Design review of the part built by this model. Coordinates are the model's own, in mm. A direction names the side the tool comes from. Coordinates: 2 decimals unless noted, no trailing zeros. Order: outer loops, then holes, each group sorted by start corner. A loop starts at its lowest first (then second) coordinate and runs counter-clockwise, first axis right, second up. Notation, with made-up numbers: (63, -21.5) - (84, -21.5) arc R23 cw to (84, 17.5) - close; hole circle Ø2 at (-33, 50.5). An arc over 180 degrees is marked (long way). Write each question's results on one line, items separated by ' | '. Start each with the question number.
```python
from build123d import *

# Parameters (mm, degrees)
F1_W      = 50.8
F1_H      = 50.8
F2_DEPTH  = 508
F5_W      = 50.8
F5_H      = 50.8
F6_DEPTH  = 50.8
F8_W      = 552.45
F8_H      = 552.45
F8_W_2    = 546.1
F8_H_2    = 546.1
F9_DEPTH  = 50.8
F10_DEPTH = 457.2
F12_DEPTH = 114.3
F13_R     = 5.08


# Not quite as in the source:
# - a pattern or mirror of a feature is missing from the dataset's text; its kind, count and spacing are read off the source's solid


with BuildPart() as f2:
    # F1 (on Top) → F2 (new body)
    with BuildSketch(Plane.XY):
        with Locations((-247.65, 247.65)):
            Rectangle(F1_W, F1_H)
    extrude(amount=F2_DEPTH)


with BuildPart() as f3_1:
    # F3: instance of F2
    add(f2.part.mirror(Plane.YZ))


with BuildPart() as f4_1:
    # F4: instance of F2
    add(f2.part.mirror(Plane.XZ))


with BuildPart() as f4_2:
    # F4: instance of F3_1
    add(f3_1.part.mirror(Plane.XZ))


with BuildPart() as f2_1:
    add(f2.part)

    add(f3_1.part)  # F6 merges F3_1

    add(f4_1.part)  # F6 merges F4_1

    add(f4_2.part)  # F6 merges F4_2
    # F5 (on face) → F6 (join)
    with BuildSketch(Plane.XY.offset(508)):
        Polygon((-273.05, 222.25), (-273.05, -273.05), (273.05, -273.05), (273.05, 273.05), (-222.25, 273.05), (-222.25, 222.25), align=None)
        with Locations((-247.65, 247.65)):
            Rectangle(F5_W, F5_H)
    extrude(amount=-F6_DEPTH)

    # F7: union 

    # F8 (on face) → F9 (join, through all)
    with BuildSketch(Plane.XY.offset(508)):
        Rectangle(F8_W, F8_H)
        Rectangle(F8_W_2, F8_H_2, mode=Mode.SUBTRACT)
    extrude(amount=-F9_DEPTH)

    # F10 (cut, through all): faces of the model
    f10_faces = [f2_1.faces().sort_by_distance(p)[0] for p in [
        (247.65, -247.65, 0),
        (247.65, 247.65, 0),
    ]]
    extrude(f10_faces, amount=-F10_DEPTH, mode=Mode.SUBTRACT)

    # F11 (on face) → F12 (join)
    with BuildSketch(Plane(origin=(0, 0, 0), x_dir=(1, 0, 0), z_dir=(0, 0, -1))):
        Polygon((-230.124, 265.176), (-265.176, 265.176), (-230.124, 230.124), align=None)
        Polygon((-230.124, 230.124), (-265.176, 265.176), (-265.176, 230.124), align=None)
    f12 = extrude(amount=F12_DEPTH)

    # F12_copies: F12 across plane
    add(f12.mirror(Plane.ZX))

    # F13
    f13_edges = [f2_1.edges().sort_by_distance(p)[0] for p in [
        (-230.124, -265.176, -57.15),
        (-265.176, -265.176, -57.15),
        (-230.124, -230.124, -57.15),
        (-265.176, -230.124, -57.15),
        (-230.124, 265.176, -57.15),
        (-265.176, 265.176, -57.15),
        (-265.176, 230.124, -57.15),
        (-230.124, 230.124, -57.15),
    ]]
    fillet(f13_edges, radius=F13_R)


solid = f2_1.part
```
(1) Take a section at A-A (z = 280). State the section outline as (x, y) points.
(2) Tool access review of faces 1 (the face through (-273.05, -247, 225)), 2 (the face through (-247, 265.176, -56)), 3 (the face through (-230.124, 247, -56)): name each direction out of +Z, -Z, +X, -X, +Y, -Y from which nothing blocks a thin tool from reaching the whole face with its end or side.
(3) Clearance check with flat-ended pins moving along their axes: pin 1 (7.5 mm diameter, centred on x = -242, z = -53, fed in from +Y); pin 2 (15 mm diameter, centred on x = -249.5, z = 193.5, fed in from +Y); pin 3 (3 mm diameter, centred on x = -178.5, y = -106, fed in from -Z). State where each tip first meets the part, or that it passes through.
(4) Take a section at B-B (y = 163.5). State the section outline as (x, z) points (3 decimals), plus the area to 3 significant figures.
(5) To check wall thickness, follow line 1 along Y through (x, z) = (-235.5, 305); line 2 along Z through (x, y) = (-212, 186.5); line 3 along X through (y, z) = (248.5, 411). State the ranges of each line that lie inside material, in increasing order. Write a range as [from, to].
Worked out:
1) outline: (-273.05, -273.05) - (-222.25, -273.05) - (-222.25, -222.25) - (-273.05, -222.25) - close; (-273.05, 222.25) - (-222.25, 222.25) - (-222.25, 273.05) - (-273.05, 273.05) - close
2) face 1: -Z, -X, +Y, -Y | face 2: -Z, +X, -X, +Y | face 3: -Z, +X, +Y, -Y
3) pin 1: y = 265.18 | pin 2: y = 273.05 | pin 3: z = 457.2
4) outline: (-276.225, 457.2) - (276.225, 457.2) - (276.225, 508) - (-276.225, 508) - close | area: 28,100 mm^2
5) line 1: [-273.05, -222.25], [222.25, 273.05] | line 2: [457.2, 508] | line 3: [-273.05, -222.25]
